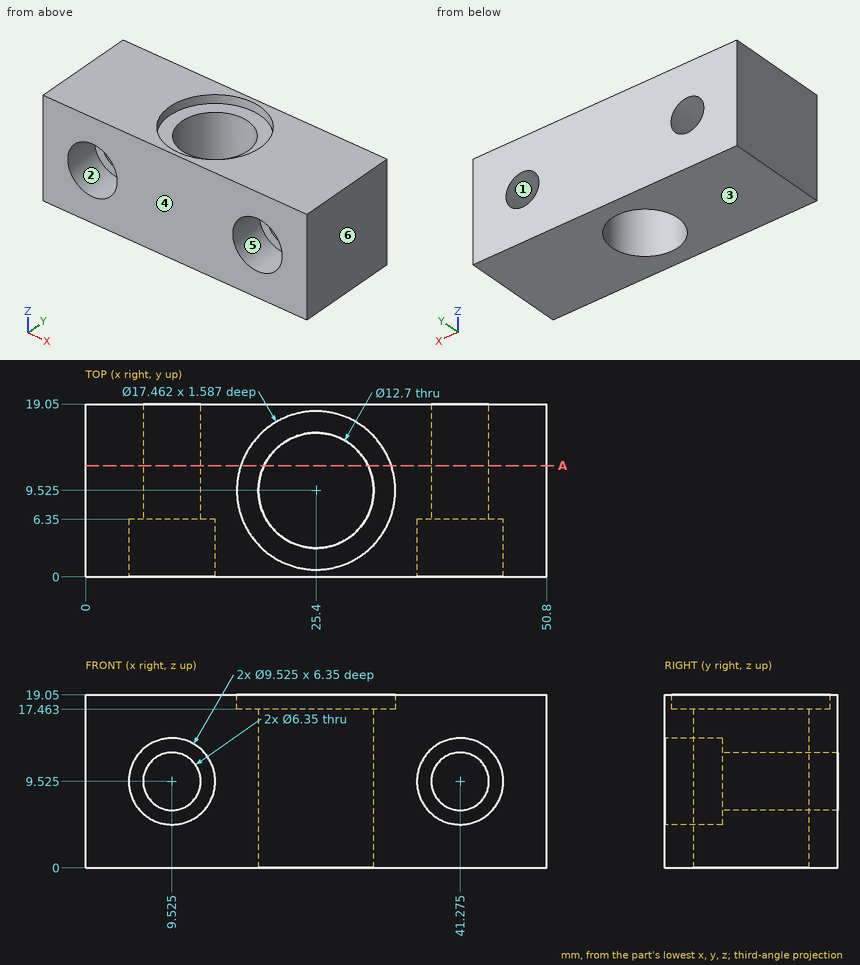
Answer from the drawing. Dimensions are ordinates in mm from the lowest x, y and z of the part. A direction names the side the tool comes from. Give positions to 0.01 mm unless a question says otherwise; leave off trailing zeros.
1) A tool of negligible diameter and unlimited length cuts with its end or side. For the marked faces 5 and 6, from which of +Z, -Z, +X, -X, +Y, -Y can it reach the whole face along a straight path? Write none if from no direction.
2) For a pull along Z with two mould halves and no side action, classify the marked faces 1, 2, 3 and 4 as pulls with the +Z half, pulls with the -Z half, needs draft (parallel to the pull), parting line crosses it, or undercut.
3) Given P1, Ø8, axis at x = 11.5, y = 16.5, coming from the -Z side; P2, Ø5, axis at x = 22.5, y = 6.5, coming from the +Z side; P3, Ø5, axis at x = 41, z = 7.5, coming from the -Y side, each flat-ended and moving along its own axis, determine where each tip first touches the part or whether it passes through.
4) Find the intervals of material crossed by L1, parallel to Y at x = 25.4, z = 18; L2, parallel to Z at x = 31, y = 13.5; L3, parallel to X at y = 8.25, z = 2.5, in increasing order.
5) Section A-A (y = 12.25) is taken. Count the separate pieces of the cut face and the enclosed holes in it, and give its area (3 significant figures).
Response:
1. face 5: -Y
1. face 6: +Z, -Z, +X, +Y, -Y
2. face 1: undercut
2. face 2: undercut
2. face 3: pulls with the -Z half
2. face 4: needs draft
3. P1: stops at z = 0
3. P2: stops at z = 17.46
3. P3: stops at y = 6.35
4. L1: y = 0 to 0.79, 18.26 to 19.05
4. L2: z = 0 to 17.46
4. L3: x = 0 to 19.18, 31.62 to 50.8
5. separate pieces: 2
5. enclosed holes: 2
5. area: 678 mm2
